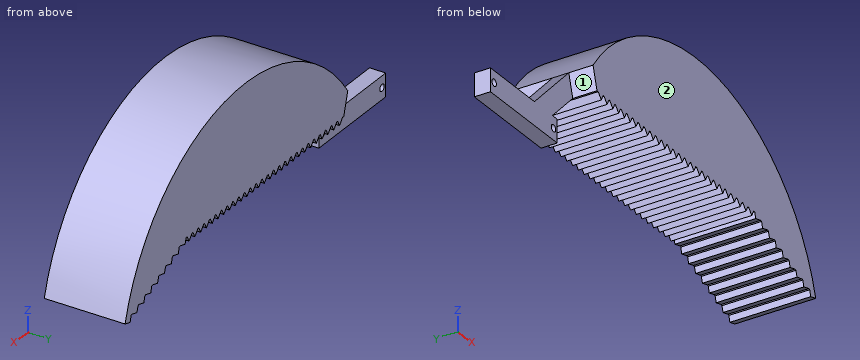
```python
from build123d import *

# Parameters (mm, degrees)
SKETCH1_W           = 45
SKETCH1_H           = 10
BOSS_EXTRUDE1_DEPTH = 7
SKETCH2_R           = 1.5
CUT_EXTRUDE1_DEPTH  = 15
BOSS_EXTRUDE2_DEPTH = 7
BOSS_EXTRUDE3_DEPTH = 17.5


with BuildPart() as part:
    # Sketch1 → Boss-Extrude1 (new body)
    with BuildSketch(Plane(origin=(0, 0, 0), x_dir=(1, 0, 0), z_dir=(0, 1, 0))):
        Rectangle(SKETCH1_W, SKETCH1_H)
    extrude(amount=BOSS_EXTRUDE1_DEPTH)

    # Sketch2 → Cut-Extrude1 (cut)
    with BuildSketch(Plane(origin=(0, 7, 0), x_dir=(1, 0, 0), z_dir=(0, 1, 0))):
        with Locations(Location((-20, 0, 0), (0, 0, 270))):
            Circle(SKETCH2_R)
        with Locations(Location((20, 0, 0), (0, 0, 270))):
            Circle(SKETCH2_R)
    extrude(amount=-CUT_EXTRUDE1_DEPTH, mode=Mode.SUBTRACT)

    # Sketch5 → Boss-Extrude2 (add)
    with BuildSketch(Plane(origin=(0, 7, 0), x_dir=(1, 0, 0), z_dir=(0, 1, 0))):
        Polygon((19.2999618, -5), (32.988821569, -18.688859769), (30.31750473, -28.162976429), (7.154528301, -5), align=None)
    extrude(amount=-BOSS_EXTRUDE2_DEPTH)

    # Sketch5_6 → Boss-Extrude3 (add, symmetric)
    with BuildSketch(Plane(origin=(0, 7, 0), x_dir=(1, 0, 0), z_dir=(0, 1, 0))):
        with BuildLine():
            Line((33.794492956, -18.688859769), (32.988821569, -18.688859769))
            Line((32.988821569, -18.688859769), (30.31750473, -28.162976429))
            ThreePointArc((30.31750473, -28.162976429), (113.686282102, -63.078391798), (180.395979402, -2.092692187))
            Line((180.395979402, -2.092692187), (177.016273904, -1.1878774))
            Line((177.016273904, -1.1878774), (176.333417559, -3.738513594))
            Line((176.333417559, -3.738513594), (175.761821244, -3.970078181))
            Line((175.761821244, -3.970078181), (172.382115747, -3.065263394))
            Line((172.382115747, -3.065263394), (171.699259402, -5.615899588))
            Line((171.699259402, -5.615899588), (171.127663087, -5.847464174))
            Line((171.127663087, -5.847464174), (167.747957589, -4.942649388))
            Line((167.747957589, -4.942649388), (167.065101244, -7.493285582))
            Line((167.065101244, -7.493285582), (166.493504929, -7.724850168))
            Line((166.493504929, -7.724850168), (163.113799431, -6.820035382))
            Line((163.113799431, -6.820035382), (162.430943086, -9.370671576))
            Line((162.430943086, -9.370671576), (161.859346771, -9.602236162))
            Line((161.859346771, -9.602236162), (158.479641274, -8.697421376))
            Line((158.479641274, -8.697421376), (157.796784929, -11.24805757))
            Line((157.796784929, -11.24805757), (157.225188614, -11.479622156))
            Line((157.225188614, -11.479622156), (153.845483116, -10.57480737))
            Line((153.845483116, -10.57480737), (153.162626771, -13.125443564))
            Line((153.162626771, -13.125443564), (152.591030456, -13.35700815))
            Line((152.591030456, -13.35700815), (149.211324958, -12.452193363))
            Line((149.211324958, -12.452193363), (148.528468613, -15.002829558))
            Line((148.528468613, -15.002829558), (147.956872298, -15.234394144))
            Line((147.956872298, -15.234394144), (144.577166801, -14.329579357))
            Line((144.577166801, -14.329579357), (143.894310456, -16.880215552))
            Line((143.894310456, -16.880215552), (143.322714141, -17.111780138))
            Line((143.322714141, -17.111780138), (139.943008643, -16.206965351))
            Line((139.943008643, -16.206965351), (139.278555847, -18.688859769))
            Line((139.278555847, -18.688859769), (138.569191128, -18.688859769))
            Line((138.569191128, -18.688859769), (137.277695253, -16.206965351))
            Line((137.277695253, -16.206965351), (135.194492956, -18.688859769))
            Line((135.194492956, -18.688859769), (134.669191128, -18.688859769))
            Line((134.669191128, -18.688859769), (133.377695253, -16.206965351))
            Line((133.377695253, -16.206965351), (131.294492956, -18.688859769))
            Line((131.294492956, -18.688859769), (130.769191128, -18.688859769))
            Line((130.769191128, -18.688859769), (129.477695253, -16.206965351))
            Line((129.477695253, -16.206965351), (127.394492956, -18.688859769))
            Line((127.394492956, -18.688859769), (126.869191128, -18.688859769))
            Line((126.869191128, -18.688859769), (125.577695253, -16.206965351))
            Line((125.577695253, -16.206965351), (123.494492956, -18.688859769))
            Line((123.494492956, -18.688859769), (122.969191128, -18.688859769))
            Line((122.969191128, -18.688859769), (121.677695253, -16.206965351))
            Line((121.677695253, -16.206965351), (119.594492956, -18.688859769))
            Line((119.594492956, -18.688859769), (119.069191128, -18.688859769))
            Line((119.069191128, -18.688859769), (117.777695253, -16.206965351))
            Line((117.777695253, -16.206965351), (115.694492956, -18.688859769))
            Line((115.694492956, -18.688859769), (115.169191128, -18.688859769))
            Line((115.169191128, -18.688859769), (113.877695253, -16.206965351))
            Line((113.877695253, -16.206965351), (111.794492956, -18.688859769))
            Line((111.794492956, -18.688859769), (111.269191128, -18.688859769))
            Line((111.269191128, -18.688859769), (109.977695253, -16.206965351))
            Line((109.977695253, -16.206965351), (107.894492956, -18.688859769))
            Line((107.894492956, -18.688859769), (107.369191128, -18.688859769))
            Line((107.369191128, -18.688859769), (106.077695253, -16.206965351))
            Line((106.077695253, -16.206965351), (103.994492956, -18.688859769))
            Line((103.994492956, -18.688859769), (103.469191128, -18.688859769))
            Line((103.469191128, -18.688859769), (102.177695253, -16.206965351))
            Line((102.177695253, -16.206965351), (100.094492956, -18.688859769))
            Line((100.094492956, -18.688859769), (99.569191128, -18.688859769))
            Line((99.569191128, -18.688859769), (98.277695253, -16.206965351))
            Line((98.277695253, -16.206965351), (96.194492956, -18.688859769))
            Line((96.194492956, -18.688859769), (95.669191128, -18.688859769))
            Line((95.669191128, -18.688859769), (94.377695253, -16.206965351))
            Line((94.377695253, -16.206965351), (92.294492956, -18.688859769))
            Line((92.294492956, -18.688859769), (91.769191128, -18.688859769))
            Line((91.769191128, -18.688859769), (90.477695253, -16.206965351))
            Line((90.477695253, -16.206965351), (88.394492956, -18.688859769))
            Line((88.394492956, -18.688859769), (87.869191128, -18.688859769))
            Line((87.869191128, -18.688859769), (86.577695253, -16.206965351))
            Line((86.577695253, -16.206965351), (84.494492956, -18.688859769))
            Line((84.494492956, -18.688859769), (83.969191128, -18.688859769))
            Line((83.969191128, -18.688859769), (82.677695253, -16.206965351))
            Line((82.677695253, -16.206965351), (80.594492956, -18.688859769))
            Line((80.594492956, -18.688859769), (80.069191128, -18.688859769))
            Line((80.069191128, -18.688859769), (78.777695253, -16.206965351))
            Line((78.777695253, -16.206965351), (76.694492956, -18.688859769))
            Line((76.694492956, -18.688859769), (76.169191128, -18.688859769))
            Line((76.169191128, -18.688859769), (74.877695253, -16.206965351))
            Line((74.877695253, -16.206965351), (72.794492956, -18.688859769))
            Line((72.794492956, -18.688859769), (72.269191128, -18.688859769))
            Line((72.269191128, -18.688859769), (70.977695253, -16.206965351))
            Line((70.977695253, -16.206965351), (68.894492956, -18.688859769))
            Line((68.894492956, -18.688859769), (68.369191128, -18.688859769))
            Line((68.369191128, -18.688859769), (67.077695253, -16.206965351))
            Line((67.077695253, -16.206965351), (64.994492956, -18.688859769))
            Line((64.994492956, -18.688859769), (64.469191128, -18.688859769))
            Line((64.469191128, -18.688859769), (63.177695253, -16.206965351))
            Line((63.177695253, -16.206965351), (61.094492956, -18.688859769))
            Line((61.094492956, -18.688859769), (60.569191128, -18.688859769))
            Line((60.569191128, -18.688859769), (59.277695253, -16.206965351))
            Line((59.277695253, -16.206965351), (57.194492956, -18.688859769))
            Line((57.194492956, -18.688859769), (56.669191128, -18.688859769))
            Line((56.669191128, -18.688859769), (55.377695253, -16.206965351))
            Line((55.377695253, -16.206965351), (53.294492956, -18.688859769))
            Line((53.294492956, -18.688859769), (52.769191128, -18.688859769))
            Line((52.769191128, -18.688859769), (51.477695253, -16.206965351))
            Line((51.477695253, -16.206965351), (49.394492956, -18.688859769))
            Line((49.394492956, -18.688859769), (48.869191128, -18.688859769))
            Line((48.869191128, -18.688859769), (47.577695253, -16.206965351))
            Line((47.577695253, -16.206965351), (45.494492956, -18.688859769))
            Line((45.494492956, -18.688859769), (44.969191128, -18.688859769))
            Line((44.969191128, -18.688859769), (43.677695253, -16.206965351))
            Line((43.677695253, -16.206965351), (41.594492956, -18.688859769))
            Line((41.594492956, -18.688859769), (41.069191128, -18.688859769))
            Line((41.069191128, -18.688859769), (39.777695253, -16.206965351))
            Line((39.777695253, -16.206965351), (37.694492956, -18.688859769))
            Line((37.694492956, -18.688859769), (37.169191128, -18.688859769))
            Line((37.169191128, -18.688859769), (35.877695253, -16.206965351))
            Line((35.877695253, -16.206965351), (33.794492956, -18.688859769))
        make_face()
    extrude(amount=BOSS_EXTRUDE3_DEPTH, both=True)


solid = part.part
```
Verification items for the finished model (mm, model axes). Face numbers are marked on the shaded views. A direction names the side the tool comes from. Coordinates: 2 decimals unless noted, no trailing zeros. Loops run counter-clockwise (first coordinate to the right, second up) from the corner with the lowest first, then second, coordinate; pieces in that order, holes last. Notation, with made-up numbers: (50, -27.5) -> (101, -27.5) arc R22 cw to (101, -16.5) -> close; hole circle Ø6 at (79.5, 38). An arc over 180 degrees is marked (long way). Put each result on its own line as item: value.
1. Section check A-A, the plane z = 37. Record the boundary of the cut face in (x, y), then the cut area to 3 significant figures.
Result set:
outline: (37.36, -10.5) -> (161.28, -10.5) -> (161.28, 24.5) -> (37.36, 24.5) -> close
area: 4,340 mm^2
2. Thickness scan on line 1 (X direction, y = 2, z = 0); line 2 (X direction, y = -5.5, z = 37); line 3 (Z direction, x = 135.5, y = -7). Record the ranges inside material, lowest first.
Result set:
line 1: x = -22.5 to -21.5, -18.5 to 18.5, 21.5 to 22.5
line 2: x = 37.36 to 161.28
line 3: z = 18.32 to 56.12
3. Gauge pin test, flat ends, axial feed: P1, Ø0.6, axis at x = 41.5, y = 6.5, coming from the -Z side; P2, Ø0.6, axis at x = 37.5, y = 9.5, coming from the -Z side; P3, Ø3.5, axis at x = 20.5, y = 3.5, coming from the +Z side. Record the tip position at first contact, or that the pin passes through.
Result set:
P1: stops at z = 18.44
P2: stops at z = 18.56
P3: stops at z = 20.1
4. Tool access check on the marked faces 1 and 2. Record the directions out of +Z, -Z, +X, -X, +Y, -Y that give a thin tool (end or side, any length) a straight path to the whole face; none if there is none.
Result set:
face 1: -Z, -X, -Y
face 2: +Z, -Z, +X, -X, -Y
5. Section check B-B, the plane z = 50.5. Record the boundary of the cut face in (x, y), then the cut area to 3 significant figures.
Result set:
outline: (53.19, -10.5) -> (145.46, -10.5) -> (145.46, 24.5) -> (53.19, 24.5) -> close
area: 3,230 mm^2
